from build123d import *

# Parameters (mm, degrees)
F0_W     = 152.4
F0_H     = 101.6
F2_DEPTH = 12.7
F1_R     = 3.81
F3_DEPTH = 25.4


with BuildPart() as f2:
    # F0 (on Front) → F2 (new body)
    with BuildSketch(Plane.XZ):
        with Locations((76.2, 50.8)):
            Rectangle(F0_W, F0_H)
    extrude(amount=F2_DEPTH)

    # F1 (on face) → F3 (cut)
    with BuildSketch(Plane.XZ):
        with Locations((12.7, 12.7)):
            Circle(F1_R)
        with Locations((12.7, 38.1)):
            Circle(F1_R)
        with Locations((12.7, 63.5)):
            Circle(F1_R)
        with Locations((12.7, 88.9)):
            Circle(F1_R)
        with Locations((38.1, 12.7)):
            Circle(F1_R)
        with Locations((38.1, 38.1)):
            Circle(F1_R)
        with Locations((38.1, 63.5)):
            Circle(F1_R)
        with Locations((38.1, 88.9)):
            Circle(F1_R)
        with Locations((63.5, 12.7)):
            Circle(F1_R)
        with Locations((63.5, 38.1)):
            Circle(F1_R)
        with Locations((63.5, 63.5)):
            Circle(F1_R)
        with Locations((63.5, 88.9)):
            Circle(F1_R)
        with Locations((88.9, 12.7)):
            Circle(F1_R)
        with Locations((88.9, 38.1)):
            Circle(F1_R)
        with Locations((88.9, 63.5)):
            Circle(F1_R)
        with Locations((88.9, 88.9)):
            Circle(F1_R)
        with Locations((114.3, 12.7)):
            Circle(F1_R)
        with Locations((114.3, 38.1)):
            Circle(F1_R)
        with Locations((114.3, 63.5)):
            Circle(F1_R)
        with Locations((114.3, 88.9)):
            Circle(F1_R)
        with Locations((139.7, 12.7)):
            Circle(F1_R)
        with Locations((139.7, 38.1)):
            Circle(F1_R)
        with Locations((139.7, 63.5)):
            Circle(F1_R)
        with Locations((139.7, 88.9)):
            Circle(F1_R)
    extrude(amount=F3_DEPTH, mode=Mode.SUBTRACT)


solid = f2.part
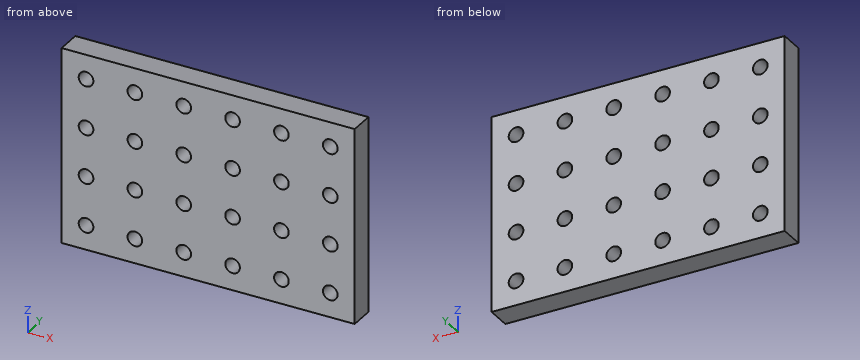
The model under review builds one solid part; all positions refer to its coordinate system, in mm. Give positions to 0.01 mm unless a question says otherwise; leave off trailing zeros. Order: outer loops, then holes, each group sorted by start corner. A loop starts at its lowest first (then second) coordinate and runs counter-clockwise, first axis right, second up. Notation, with made-up numbers: M 70.5,11.5 L 125.5,11.5 A33 ccw 125.5,40.5 Z; hole C 56,70.5 d2. An arc over 180 degrees is marked long. Use one line per item in the form item = value. Start each with the question number.
Item 1: To check wall thickness, follow line 1 along Z through (x, y) = (89, -2.25); line 2 along Z through (x, y) = (40.5, -7.5). State the ranges of each line that lie inside material, in increasing order. Write a range as from..to.
Item 2: We need section C-C on y = -7.25. Give the number of separate pieces and of enclosed holes in the cut face, plus the area to 3 significant figures.
Item 3: We need section B-B on z = 38.1. Give the boundary of the cut face in (x, y).
Item 4: We need section A-A on x = 38.1. Give the boundary of the cut face in (y, z), plus the area to 3 significant figures.
Completed:
q1.line_1 = 0..8.89, 16.51..34.29, 41.91..59.69, 67.31..85.09, 92.71..101.6
q1.line_2 = 0..9.74, 15.66..35.14, 41.06..60.54, 66.46..85.94, 91.86..101.6
q2.separate_pieces = 1
q2.enclosed_holes = 24
q2.area = 14,400 mm²
q3.outline = M 0,-12.7 L 8.89,-12.7 L 8.89,0 L 0,0 Z; M 16.51,-12.7 L 34.29,-12.7 L 34.29,0 L 16.51,0 Z; M 41.91,-12.7 L 59.69,-12.7 L 59.69,0 L 41.91,0 Z; M 67.31,-12.7 L 85.09,-12.7 L 85.09,0 L 67.31,0 Z; M 92.71,-12.7 L 110.49,-12.7 L 110.49,0 L 92.71,0 Z; M 118.11,-12.7 L 135.89,-12.7 L 135.89,0 L 118.11,0 Z; M 143.51,-12.7 L 152.4,-12.7 L 152.4,0 L 143.51,0 Z
q4.outline = M -12.7,0 L 0,0 L 0,8.89 L -12.7,8.89 Z; M -12.7,16.51 L 0,16.51 L 0,34.29 L -12.7,34.29 Z; M -12.7,41.91 L 0,41.91 L 0,59.69 L -12.7,59.69 Z; M -12.7,67.31 L 0,67.31 L 0,85.09 L -12.7,85.09 Z; M -12.7,92.71 L 0,92.71 L 0,101.6 L -12.7,101.6 Z
q4.area = 903 mm²
